Verification items for the finished model (mm, model axes). A direction names the side the tool comes from. Round coordinates to 2 decimals unless told otherwise and drop trailing zeros. Write each loop counter-clockwise with the first axis right and the second up, starting at its lowest first coordinate (ties: lowest second). Pieces come first, ordered by that corner, then holes.
from build123d import *

# Parameters (mm, degrees)
SKETCH1_R           = 6
SKETCH1_R_2         = 8.5
BOSS_EXTRUDE1_DEPTH = 8
FILLET1_R           = 5


with BuildPart() as part:
    # Sketch1 → Boss-Extrude1 (new body)
    with BuildSketch(Plane.XY):
        with BuildLine():
            ThreePointArc((12.5, -13.638181697), (0, 18.5), (-12.5, -13.638181697))
            Line((-12.5, -13.638181697), (-12.5, -23))
            ThreePointArc((-12.5, -23), (-6.5, -35), (-12.5, -47))
            Line((-12.5, -47), (-12.5, -152.456671403))
            Line((-12.5, -152.456671403), (0, -152.456671403))
            ThreePointArc((0, -152.456671403), (32.019441409, -179.184193262), (11.444366088, -215.464647068))
            ThreePointArc((11.444366088, -215.464647068), (-18.29086587, -232.773846738), (15.239317045, -240.488718511))
            ThreePointArc((15.239317045, -240.488718511), (57.52601951, -183.58870793), (12.5, -128.830749818))
            Line((12.5, -128.830749818), (12.5, -47))
            ThreePointArc((12.5, -47), (6.5, -35), (12.5, -23))
            Line((12.5, -23), (12.5, -13.638181697))
        make_face()
        with BuildLine():
            ThreePointArc((8.333859781, -228.327642037), (8.458362966, -229.159704854), (8.5, -230))
            ThreePointArc((8.5, -230), (-8.458362966, -230.840295146), (8.333859781, -228.327642037))
        make_face(mode=Mode.SUBTRACT)
        with BuildLine():
            ThreePointArc((0, -146.456671403), (-0.878679656, -148.577991747), (-3, -149.456671403))
            Line((-3, -149.456671403), (-6.5, -149.456671403))
            ThreePointArc((-6.5, -149.456671403), (-8.621320344, -148.577991747), (-9.5, -146.456671403))
            Line((-9.5, -146.456671403), (-9.5, -136.26051898))
            ThreePointArc((-9.5, -136.26051898), (-9.397777479, -135.484061845), (-9.098076211, -134.76051898))
            Line((-9.098076211, -134.76051898), (-6.366025404, -130.028468173))
            ThreePointArc((-6.366025404, -130.028468173), (-5.267949192, -128.930391962), (-3.767949192, -128.528468173))
            Line((-3.767949192, -128.528468173), (1.5, -128.528468173))
            ThreePointArc((1.5, -128.528468173), (3.621320344, -129.407147829), (4.5, -131.528468173))
            Line((4.5, -131.528468173), (4.5, -136.858595192))
            ThreePointArc((4.5, -136.858595192), (4.397777479, -137.635052327), (4.098076211, -138.358595192))
            Line((4.098076211, -138.358595192), (0.401923789, -144.76051898))
            ThreePointArc((0.401923789, -144.76051898), (0.102222521, -145.484061845), (0, -146.26051898))
            Line((0, -146.26051898), (0, -146.456671403))
        make_face(mode=Mode.SUBTRACT)
        with BuildLine():
            ThreePointArc((43.461464413, -168.466666667), (46.5, -185), (43.461464413, -201.533333333))
            ThreePointArc((43.461464413, -201.533333333), (41.526148356, -202.401982723), (40.657498967, -200.466666667))
            ThreePointArc((40.657498967, -200.466666667), (43.5, -185), (40.657498967, -169.533333333))
            ThreePointArc((40.657498967, -169.533333333), (41.526148356, -167.598017277), (43.461464413, -168.466666667))
        make_face(mode=Mode.SUBTRACT)
        with BuildLine():
            ThreePointArc((7.5, -119.456671403), (0, -126.956671403), (-7.5, -119.456671403))
            Line((-7.5, -119.456671403), (-7.5, -80.654914144))
            ThreePointArc((-7.5, -80.654914144), (-7.485723324, -80.000623333), (-7.442920471, -79.347578002))
            Line((-7.442920471, -79.347578002), (-6.756300289, -71.499473409))
            ThreePointArc((-6.756300289, -71.499473409), (-6.133334804, -70.658889988), (-5.101807809, -70.833871534))
            ThreePointArc((-5.101807809, -70.833871534), (0, -72.75), (5.101807809, -70.833871534))
            ThreePointArc((5.101807809, -70.833871534), (6.133334804, -70.658889988), (6.756300289, -71.499473409))
            Line((6.756300289, -71.499473409), (7.442920471, -79.347578002))
            ThreePointArc((7.442920471, -79.347578002), (7.485723324, -80.000623333), (7.5, -80.654914144))
            Line((7.5, -80.654914144), (7.5, -119.456671403))
        make_face(mode=Mode.SUBTRACT)
        with Locations((0, -65)):
            Circle(SKETCH1_R, mode=Mode.SUBTRACT)
        with BuildLine():
            Line((-8.421524221, -21), (-10.243145112, -6.164088407))
            ThreePointArc((-10.243145112, -6.164088407), (-9.913994973, -5.631910779), (-9.323094991, -5.837799225))
            ThreePointArc((-9.323094991, -5.837799225), (0, -11), (9.323094991, -5.837799225))
            ThreePointArc((9.323094991, -5.837799225), (9.913994973, -5.631910779), (10.243145112, -6.164088407))
            Line((10.243145112, -6.164088407), (8.421524221, -21))
            add(Edge.make_bspline(
                [(5.648127088, -47.738954624), (-0.877088936, -33.717206836), (8.421524221, -21)],
                knots=[0, 0, 0, 1, 1, 1], degree=2))
            Line((5.648127088, -47.738954624), (6.09481015, -52.844565385))
            ThreePointArc((6.09481015, -52.844565385), (6.132863169, -53.716122812), (6.09481015, -54.58768024))
            Line((6.09481015, -54.58768024), (5.737570571, -58.670947304))
            ThreePointArc((5.737570571, -58.670947304), (5.433124471, -59.088345781), (4.921929391, -59.013589467))
            ThreePointArc((4.921929391, -59.013589467), (0, -57.25), (-4.921929391, -59.013589467))
            ThreePointArc((-4.921929391, -59.013589467), (-5.433124471, -59.088345781), (-5.737570571, -58.670947304))
            Line((-5.737570571, -58.670947304), (-6.09481015, -54.58768024))
            ThreePointArc((-6.09481015, -54.58768024), (-6.132863169, -53.716122812), (-6.09481015, -52.844565385))
            Line((-6.09481015, -52.844565385), (-5.648127088, -47.738954624))
            add(Edge.make_bspline(
                [(-5.648127088, -47.738954624), (0.877088936, -33.717206836), (-8.421524221, -21)],
                knots=[0, 0, 0, 1, 1, 1], degree=2))
        make_face(mode=Mode.SUBTRACT)
        Circle(SKETCH1_R_2, mode=Mode.SUBTRACT)
    extrude(amount=BOSS_EXTRUDE1_DEPTH)

    # Fillet1
    fillet1_edges = [part.edges().sort_by_distance(p)[0] for p in [
        (11.444366088, -215.464647068, 4),
        (-12.5, -152.456671403, 4),
        (-12.5, -13.638181697, 4),
        (12.5, -13.638181697, 4),
        (12.5, -128.830749818, 4),
        (15.239317045, -240.488718511, 4),
    ]]
    fillet(fillet1_edges, radius=FILLET1_R)


solid = part.part
Q1. Depth check by flat-ended pin: P1, Ø1, axis at y = -84, z = 5.5, coming from the -X side; P2, Ø2.5, axis at y = -89, z = 4, coming from the +X side; P3, Ø4, axis at x = -4.5, z = 2.5, coming from the +Y side; P4, Ø13.5, axis at x = 0, y = 0, coming from the +Z side. Enter the tip coordinate at first touch or a pass-through.
Recorded:
P1: stops at x = -12.5
P2: stops at x = 12.5
P3: stops at y = 18.33
P4: passes through
Q2. Sectioned sample at C-C (z = 6.5). Give the number of separate pieces and of enclosed holes in the cut face, plus the area to 3 significant figures.
Recorded:
separate pieces: 1
enclosed holes: 7
area: 5,860 mm2
Q3. Release check for a two-part mould opening along Y. For faces 4 (the flat face through (9.345, -13.478, 3.944)), 5 (the cylindrical face through (0, -11, 4)) record: released by +Y, released by -Y, zero draft, split by the parting line, or undercut.
Recorded:
face 4: undercut
face 5: undercut
Q4. Tool access check on faces 1 (the flat face through (-12.5, -19, 4)), 2 (the cylindrical face through (13.473, -127.919, 4.056)), 3 (the flat face through (-7.5, -100, 4)). Record the directions out of +Z, -Z, +X, -X, +Y, -Y that give a thin tool (end or side, any length) a straight path to the whole face; none if there is none.
Recorded:
face 1: +Z, -Z, -X
face 2: +Z, -Z, +X
face 3: +Z, -Z
Q5. Sectioned sample at B-B (y = 0). Enter the section's corners in (x, z).
Recorded:
outline: (-18.5, 0) - (-8.5, 0) - (-8.5, 8) - (-18.5, 8) - close; (8.5, 0) - (18.5, 0) - (18.5, 8) - (8.5, 8) - close
Q6. Material ranges on line 1 along X through (y, z) = (-81, 5.25); line 2 along X through (y, z) = (-49, 2.25); line 3 along Y through (x, z) = (21.5, 1.75), recorded low to high.
Recorded:
line 1: x = -12.5 to -7.5, 7.5 to 12.5
line 2: x = -12.5 to -5.76, 5.76 to 12.5
line 3: y = -238.38 to -209.43, -160.57 to -131.62
Q7. Sectioned sample at A-A (y = -65). Enter the section's corners in (x, z), plus the area to 3 significant figures.
Recorded:
outline: (-12.5, 0) - (-6, 0) - (-6, 8) - (-12.5, 8) - close; (6, 0) - (12.5, 0) - (12.5, 8) - (6, 8) - close
area: 104 mm2
